Read the model definition and answer for the solid it produces. Units are mm, in the model's axes. A direction names the side the tool comes from. Coordinates: 2 decimals unless noted, no trailing zeros. Write each loop counter-clockwise with the first axis right and the second up, starting at its lowest first coordinate (ties: lowest second). Pieces come first, ordered by that corner, then holes. Notation, with made-up numbers: M 64.25,-19.5 L 123.25,-19.5 A21 ccw 123.25,-12.5 Z; hole C -15,16 d1. An arc over 180 degrees is marked long. Write item = value, one per line.
from build123d import *

# Parameters (mm, degrees)
BOSS_EXTRUDE1_DEPTH = 60
FILLET1_R           = 1
BOSS_EXTRUDE2_DEPTH = 3


with BuildPart() as part:
    # Sketch2 → Boss-Extrude1 (new body)
    with BuildSketch(Plane(origin=(0, 0, 0), x_dir=(0, 0, -1), z_dir=(1, 0, 0))):
        Polygon((0, 0), (0, 23), (10.33, 23), (10.33, 20), (5.33, 4.995680218), (25.33, 4.995680218), (20.33, 20), (20.33, 23), (30.66, 23), (30.66, 0), align=None)
    extrude(amount=BOSS_EXTRUDE1_DEPTH)

    # Fillet1
    fillet1_edges = [part.edges().sort_by_distance(p)[0] for p in [
        (0, 11.5, 0),
        (0, 11.5, -30.66),
        (0, 0, -15.33),
        (30, 0, 0),
        (30, 23, 0),
        (30, 23, -30.66),
        (30, 0, -30.66),
        (60, 11.5, 0),
        (60, 0, -15.33),
        (60, 11.5, -30.66),
    ]]
    fillet(fillet1_edges, radius=FILLET1_R)

    # Sketch3 → Boss-Extrude2 (add)
    with BuildSketch(Plane.ZY):
        Polygon((-20.33, 23), (-10.33, 23), (-10.33, 20), (-5.33, 4.995680218), (-25.33, 4.995680218), (-20.33, 20), align=None)
    extrude(amount=-BOSS_EXTRUDE2_DEPTH)


solid = part.part
Item 1: For a pull along Z with two mould halves and no side action, classify faces 4 (the face through (31, 21, -20.33)), 5 (the face through (30, 23, -22)), 6 (the face through (31.101, 12.393, -22.865)), 7 (the face through (30, 12, -30.66)) as released by +Z, released by -Z, zero draft, split by the parting line, or undercut.
Worked answers:
face_4 = undercut
face_5 = zero draft
face_6 = undercut
face_7 = released by -Z
Item 2: Consider line 1 along Y through (x, z) = (41, -12); line 2 along Z through (x, y) = (40.5, 9.25); line 3 along X through (y, z) = (12, -20). Determine where each line is inside the solid, lowest interval first. Write a range as from..to.
Worked answers:
line_1 = 0..5
line_2 = -30.66..-23.91, -6.75..0
line_3 = 0..3
Item 3: Flat-ended cylindrical pins translate along their axes: pin 1 (5.5 mm diameter, centred on y = 13, z = -14.5, fed in from +X); pin 2 (8 mm diameter, centred on x = 40.5, z = -15.5, fed in from +Y). Find the tip coordinate at first contact, or state that the pin passes through.
Worked answers:
pin_1 = 3
pin_2 = 5
Item 4: Find section D-D (z = -6.5). Determine the outline of the cut face in (x, y), and give its area (3 significant figures).
Worked answers:
outline = M 0,1 A1 ccw 1,0 L 59,0 A1 ccw 60,1 L 60,5 L 3,5 L 3,8.51 L 60,8.51 L 60,23 L 0,23 Z
area = 1,180 mm²
Item 5: Find section A-A (z = -15). Determine the outline of the cut face in (x, y), and give its area (3 significant figures).
Worked answers:
outline = M 0,1 A1 ccw 1,0 L 59,0 A1 ccw 60,1 L 60,5 L 3,5 L 3,23 L 0,23 Z
area = 353 mm²
Item 6: Find section B-B (y = 10). Determine the outline of the cut face in (x, z), and give its area (3 significant figures).
Worked answers:
outline = M 0,-29.66 A1 ccw 1,-30.66 L 59,-30.66 A1 ccw 60,-29.66 L 60,-23.66 L 3,-23.66 L 3,-7 L 60,-7 L 60,-1 A1 ccw 59,0 L 1,0 A1 ccw 0,-1 Z
area = 889 mm²
Item 7: Find section C-C (x = 50). Determine the outline of the cut face in (y, z), and give its area (3 significant figures).
Worked answers:
outline = M 0,-29.66 A1 ccw 1,-30.66 L 22,-30.66 A1 ccw 23,-29.66 L 23,-20.33 L 20,-20.33 L 5,-25.33 L 5,-5.33 L 20,-10.33 L 23,-10.33 L 23,-1 A1 ccw 22,0 L 1,0 A1 ccw 0,-1 Z
area = 449 mm²
Item 8: Which of the six approach directions +Z, -Z, +X, -X, +Y, -Y give full straight-line access (tool end or side, diameter ignored) to faces 1 (the face through (31, 22, -10.33)), 2 (the face through (30, 11, 0)), 3 (the face through (3, 12, -15))?
Worked answers:
face_1 = +X, +Y
face_2 = +Z, +X, -X, +Y, -Y
face_3 = +X
